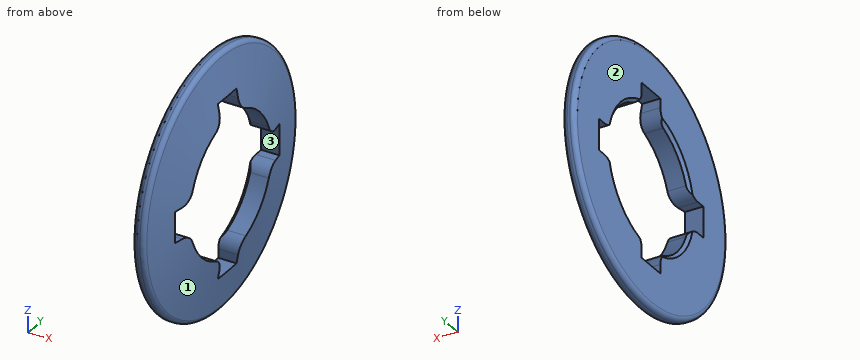
from build123d import *

# Parameters (mm, degrees)
F3_DEPTH = 25
F4_SIZE  = 1
F5_R     = 5
F6_R     = 1.5


with BuildPart() as f1:
    # F0 (on Front) → F1 (revolve)
    with BuildSketch(Plane.XZ):
        Polygon((0, 22), (-3.3502126335, 41), (-7, 41), (-7, 22), align=None)
    revolve(axis=Axis((-11.3754170015, 0, 0), (-1, 0, 0)))

    # F2 (on Right) → F3 (cut)
    with BuildSketch(Plane.YZ):
        with BuildLine():
            Line((5, 21.4242852856), (5, 28))
            Line((5, 28), (0, 28))
            Line((0, 28), (-5, 28))
            Line((-5, 28), (-5, 21.4242852856))
            ThreePointArc((-5, 21.4242852856), (0, 22), (5, 21.4242852856))
        make_face()
        with BuildLine():
            Line((-27.9999999801, -5.0000001113), (-21.4242852658, -5.0000000852))
            ThreePointArc((-21.4242852658, -5.0000000852), (-22, -8.74e-08), (-21.4242853055, 4.9999999148))
            Line((-21.4242853055, 4.9999999148), (-28.0000000199, 4.9999998887))
            Line((-28.0000000199, 4.9999998887), (-28, -1.113e-07))
            Line((-28, -1.113e-07), (-27.9999999801, -5.0000001113))
        make_face()
        with BuildLine():
            Line((5.0000002226, -27.9999999603), (5.0000001703, -21.4242852459))
            ThreePointArc((5.0000001703, -21.4242852459), (1.749e-07, -22), (-4.9999998297, -21.4242853254))
            Line((-4.9999998297, -21.4242853254), (-4.9999997774, -28.0000000397))
            Line((-4.9999997774, -28.0000000397), (2.226e-07, -28))
            Line((2.226e-07, -28), (5.0000002226, -27.9999999603))
        make_face()
        with BuildLine():
            Line((27.9999999404, 5.0000003339), (21.424285226, 5.0000002555))
            ThreePointArc((21.424285226, 5.0000002555), (22, 2.623e-07), (21.4242853453, -4.9999997445))
            Line((21.4242853453, -4.9999997445), (28.0000000596, -4.9999996661))
            Line((28.0000000596, -4.9999996661), (28, 3.339e-07))
            Line((28, 3.339e-07), (27.9999999404, 5.0000003339))
        make_face()
    extrude(amount=-F3_DEPTH, mode=Mode.SUBTRACT)

    # F4
    f4_edges = [f1.edges().sort_by_distance(p)[0] for p in [
        (-7, 15.556349, 15.556349),
        (-7, -15.556349, 15.556349),
        (-7, -15.556349, -15.556349),
        (-7, 15.556349, -15.556349),
    ]]
    chamfer(f4_edges, length=F4_SIZE)

    # F5
    f5_edges = [f1.edges().sort_by_distance(p)[0] for p in [
        (-3, -5, -21.424285),
        (-3, 5, -21.424285),
        (-3, 21.424285, -5),
        (-3, 21.424285, 5),
        (-3, 5, 21.424285),
        (-3, -5, 21.424285),
        (-3, -21.424285, 5),
        (-3, -21.424285, -5),
    ]]
    fillet(f5_edges, radius=F5_R)

    # F6
    f6_edges = [f1.edges().sort_by_distance(p)[0] for p in [
        (-3.350213, 0, -41),
        (-7, 0, -41),
    ]]
    fillet(f6_edges, radius=F6_R)


solid = f1.part
Verification items for the finished model (mm, model axes). Face numbers are marked on the shaded views. Round coordinates to 2 decimals unless told otherwise and drop trailing zeros. Use a Markdown table: item, result. Add a question column.
1. Gauge pin test, flat ends, axial feed: pin 1 (4 mm diameter, centred on y = 20, z = -23, fed in from +X); pin 2 (3 mm diameter, centred on x = -3, y = -0.5, fed in from -Z); pin 3 (3 mm diameter, centred on x = -5, z = 27, fed in from +Y). Record the tip position at first contact, or that the pin passes through.
2. Thickness scan on probe 1 along Z at (x, y) = (-5.25, 0); probe 2 along Z at (x, y) = (-3.5, 7.5); probe 3 along Y at (x, z) = (-5.25, 27). Record the ranges inside material, lowest first. Write a range as [from, to].
3. Release check for a two-part mould opening along Z. For the marked faces 1, 2 and 3 record: released by +Z, released by -Z, zero draft, split by the parting line, or undercut.
Checks:
| question | item | result |
|---|---|---|
| 1 | pin 1 | stops at x = -1.14 |
| 1 | pin 2 | stops at z = -40.99 |
| 1 | pin 3 | stops at y = 32.11 |
| 2 | probe 1 | z = [-41, -28], [28, 41] |
| 2 | probe 2 | z = [-39.81, -20.75], [20.75, 39.81] |
| 2 | probe 3 | y = [-30.85, -5], [5, 30.85] |
| 3 | face 1 | split by the parting line |
| 3 | face 2 | zero draft |
| 3 | face 3 | undercut |
